```python
from build123d import *
from build123d.topology import SkipClean

# Parameters (mm, degrees)
SKETCH_2_R               = 25
EXTRUDE_1_DEPTH          = 9
SKETCH_3_R               = 14
SKETCH_3_R_2             = 5.5
CUT_EXTRUDE_1_DEPTH      = 3
CUT_EXTRUDE_3_DEPTH      = 13
SKETCH_6_R               = 2
CUT_EXTRUDE_4_DEPTH      = 5
CUT_EXTRUDE_5_DEPTH      = 20
PATTERN_CIRCULAR_1_COUNT = 8
SKETCH_8_R               = 5.5
CUT_EXTRUDE_6_DEPTH      = 3


with BuildPart() as part:
    # 草图2 → 凸台-拉伸1 (new, symmetric)
    with BuildSketch(Plane.XY):
        Circle(SKETCH_2_R)
    extrude(amount=EXTRUDE_1_DEPTH, both=True)

    # 草图3 → 切除-拉伸1 (cut)
    with BuildSketch(Plane.XY.offset(9)):
        Circle(SKETCH_3_R)
        Circle(SKETCH_3_R_2, mode=Mode.SUBTRACT)
    cut_extrude_1 = extrude(amount=-CUT_EXTRUDE_1_DEPTH, mode=Mode.SUBTRACT)

    # 镜向1: 切除-拉伸1 across plane
    add(cut_extrude_1.mirror(Plane.XY), mode=Mode.SUBTRACT)

    # 草图5 → 切除-拉伸3 (cut)
    with BuildSketch(Plane.XY.offset(9)):
        Polygon((3.25, -1.876388375), (3.25, 1.876388375), (0, 3.75277675), (-3.25, 1.876388375), (-3.25, -1.876388375), (0, -3.75277675), align=None)
    extrude(amount=-CUT_EXTRUDE_3_DEPTH, mode=Mode.SUBTRACT)

    # 草图6 → 切除-拉伸4 (cut)
    with BuildSketch(Plane(origin=(0, 0, -9), x_dir=(-1, 0, 0), z_dir=(0, 0, -1))):
        Circle(SKETCH_6_R)
    extrude(amount=-CUT_EXTRUDE_4_DEPTH, mode=Mode.SUBTRACT)

    # 草图7 → 切除-拉伸5 (cut)
    with BuildSketch(Plane(origin=(0, 0, -6), x_dir=(-1, 0, 0), z_dir=(0, 0, -1))):
        with BuildLine():
            Line((0.750176034, 13.979886835), (0.750176034, 5.448599446))
            ThreePointArc((0.750176034, 5.448599446), (2.104758878, 5.081337429), (3.322287055, 4.383196177))
            Line((3.322287055, 4.383196177), (9.35481822, 10.415727342))
            ThreePointArc((9.35481822, 10.415727342), (5.357568053, 12.934313455), (0.750176034, 13.979886835))
        make_face()
    cut_extrude_5 = extrude(amount=-CUT_EXTRUDE_5_DEPTH, mode=Mode.SUBTRACT)

    # 阵列(圆周)1: 切除-拉伸5 ×8 about axis
    with SkipClean():  # the faces are left unmerged after this step: merging them gives an invalid solid
        pattern_circular_1_axis = Axis((0, 0, 0), (0, 0, 1))
        for i in range(1, PATTERN_CIRCULAR_1_COUNT):
            add(cut_extrude_5.rotate(pattern_circular_1_axis, i * 360 / PATTERN_CIRCULAR_1_COUNT), mode=Mode.SUBTRACT)

    # 草图8 → 切除-拉伸6 (cut)
    with SkipClean():  # the faces are left unmerged after this step: merging them gives an invalid solid
        with BuildSketch(Plane(origin=(0, 0, -9), x_dir=(-1, 0, 0), z_dir=(0, 0, -1))):
            with Locations(Location((0, 0, 0), (0, 0, 180))):
                Circle(SKETCH_8_R)
        extrude(amount=-CUT_EXTRUDE_6_DEPTH, mode=Mode.SUBTRACT)


solid = part.part
```
Check sheet for the modelled part. Datum: model origin and axes. Units: mm. A direction names the side the tool comes from. Coordinates: 2 decimals unless noted, no trailing zeros. Loops run counter-clockwise (first coordinate to the right, second up) from the corner with the lowest first, then second, coordinate; pieces in that order, holes last.
1) Sectioned sample at B-B (x = 12). Record the boundary of the cut face in (y, z), and give its area (3 significant figures).
2) Sectioned sample at A-A (z = 7). Record the boundary of the cut face in (x, y), and give its area (3 significant figures).
3) Sectioned sample at C-C (z = -7.25). Record the boundary of the cut face in (x, y), and give its area (3 significant figures).
4) Gauge pin test, flat ends, axial feed: pin 1 (4.5 mm diameter, centred on x = 8, z = 3, fed in from +Y); pin 2 (8 mm diameter, centred on x = 11, z = 6, fed in from -Y); pin 3 (5.5 mm diameter, centred on x = -5.5, y = -6, fed in from -Z). Record the tip position at first contact, or that the pin passes through.
5) Access from +Z, -Z, +X, -X, +Y, -Y to the whole of each face (thin tool, end or side, straight path). Record for faces 1 (the face through (-10, 0, 6)), 2 (the face through (6.3, -7.36, -0.08)).
6) Sectioned sample at D-D (y = -19.5). Record the boundary of the cut face in (x, z), and give its area (3 significant figures).
7) Material ranges on probe 1 along Y at (x, z) = (0, -4.4); probe 2 along X at (y, z) = (-8, -4.25); probe 3 along X at (y, z) = (-12, -0.25), recorded low to high.
8) Release check for a two-part mould opening along Y. For faces 3 (the face through (-1.6, 2.83, 2.59)), 4 (the face through (7, -7, 6)), 5 (the face through (2, 3, 9)) record: released by +Y, released by -Y, zero draft, split by the parting line, or undercut.
Check sheet entries:
1. outline: (-21.93, -9) - (-7.21, -9) - (-7.21, 9) - (-21.93, 9) - close; (-0.75, -6) - (0.75, -6) - (0.75, 6) - (-0.75, 6) - close; (7.21, -9) - (21.93, -9) - (21.93, 9) - (7.21, 9) - close
1. area: 548 mm2
2. outline: circle Ø50 at (0, 0); circle Ø11 at (0, 0); hole circle Ø28 at (0, 0); hole (-3.25, -1.88) - (0, -3.75) - (3.25, -1.88) - (3.25, 1.88) - (0, 3.75) - (-3.25, 1.88) - close
2. area: 1,410 mm2
3. outline: circle Ø50 at (0, 0); hole circle Ø28 at (0, 0)
3. area: 1,350 mm2
4. pin 1: stops at y = 24.33
4. pin 2: stops at y = -24
4. pin 3: stops at z = -6
5. face 1: +Z
5. face 2: +Z, -Z
6. outline: (-15.64, -9) - (15.64, -9) - (15.64, 9) - (-15.64, 9) - close
6. area: 563 mm2
7. probe 1: y = -25 to -2, 2 to 25
7. probe 2: x = -23.69 to -11.49, -9.06 to -6.94, -0.75 to 0.75, 6.94 to 9.06, 11.49 to 23.69
7. probe 3: x = -21.93 to -7.21, -0.75 to 0.75, 7.21 to 21.93
8. face 3: undercut
8. face 4: undercut
8. face 5: zero draft
